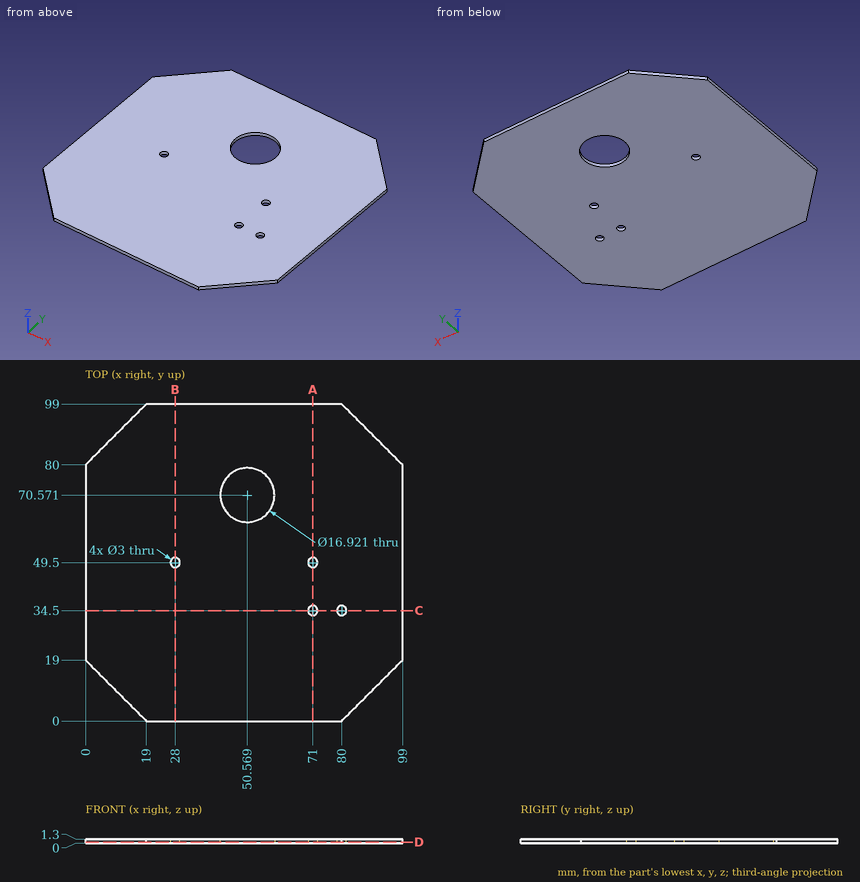
Geometry: see drawing. Coordinates: mm, zero at the bounding-box minimum. Round coordinates to 2 decimals unless told otherwise and drop trailing zeros. Loops run counter-clockwise (first coordinate to the right, second up) from the corner with the lowest first, then second, coordinate; pieces in that order, holes last. Notation, with made-up numbers: (-16.75, 74.5) -> (10.25, 74.5) arc R22 cw to (10.25, 113.5) -> close; hole circle Ø9 at (89, 25). An arc over 180 degrees is marked (long way). Write each question's results on one line, items separated by ' | '.
1. Section C-C (y = 34.5). Return loops of the section in (x, z).
Geometry results:
outline: (0, 0) -> (69.5, 0) -> (69.5, 1.3) -> (0, 1.3) -> close; (72.5, 0) -> (78.5, 0) -> (78.5, 1.3) -> (72.5, 1.3) -> close; (81.5, 0) -> (99, 0) -> (99, 1.3) -> (81.5, 1.3) -> close
2. Ray query, line 1 (Y direction, x = 71, z = 0.6); line 2 (Y direction, x = 28, z = 0.7); line 3 (X direction, y = 71, z = 1.25). Return the intervals inside material, ascending. Write a range as from..to.
Geometry results:
line 1: 0..33, 36..48, 51..99 | line 2: 0..48, 51..99 | line 3: 0..42.12, 59.02..99
3. Section A-A (x = 71). Return loops of the section in (y, z), and give its area (3 significant figures).
Geometry results:
outline: (0, 0) -> (33, 0) -> (33, 1.3) -> (0, 1.3) -> close; (36, 0) -> (48, 0) -> (48, 1.3) -> (36, 1.3) -> close; (51, 0) -> (99, 0) -> (99, 1.3) -> (51, 1.3) -> close | area: 121 mm2
4. Section B-B (x = 28). Return loops of the section in (y, z), and give its area (3 significant figures).
Geometry results:
outline: (0, 0) -> (48, 0) -> (48, 1.3) -> (0, 1.3) -> close; (51, 0) -> (99, 0) -> (99, 1.3) -> (51, 1.3) -> close | area: 125 mm2
5. Section D-D (z = 0.3). Return loops of the section in (x, y).
Geometry results:
outline: (0, 19) -> (19, 0) -> (80, 0) -> (99, 19) -> (99, 80) -> (80, 99) -> (19, 99) -> (0, 80) -> close; hole circle Ø3 at (28, 49.5); hole circle Ø16.92 at (50.57, 70.57); hole circle Ø3 at (71, 34.5); hole circle Ø3 at (71, 49.5); hole circle Ø3 at (80, 34.5)
